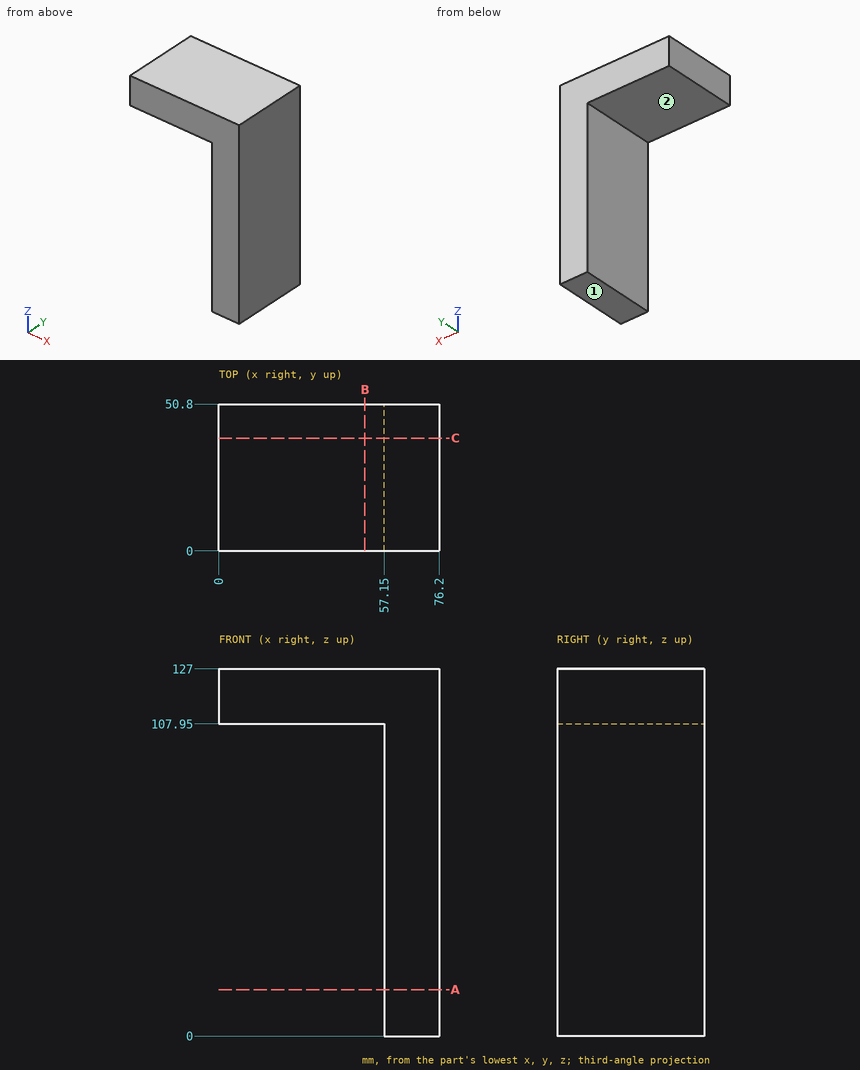
Answer from the drawing. Dimensions are ordinates in mm from the lowest x, y and z of the part. A direction names the side the tool comes from. Give positions to 0.01 mm unless a question says otherwise; leave off trailing zeros. Order: outer loops, then holes, each group sorted by start corner. A loop starts at its lowest first (then second) coordinate and runs counter-clockwise, first axis right, second up. Notation, with made-up numbers: (48.25, 43) -> (55.25, 43) arc R30 ccw to (55.25, 68) -> close; hole circle Ø2 at (73, 75.25). An arc over 180 degrees is marked (long way). One line per item, written item: value. Start each with the question number.
(1) The part is cut by section A-A (z = 16). Determine the outline of the cut face in (x, y), and give its area (3 significant figures).
(2) A tool of negligible diameter and unlimited length cuts with its end or side. For the marked faces 1 and 2, from which of +Z, -Z, +X, -X, +Y, -Y can it reach the whole face along a straight path? Write none if from no direction.
(3) Straight lines are drawn through the part: L1, parallel to X at y = 5, z = 89.5; L2, parallel to Z at x = 45, y = 8.5. For each, find the intervals that lie inside material, in ascending order.
(4) A flat-ended cylindrical pin translates along its axis: P1, Ø3, axis at y = 15.5, z = 17.5, coming from the -X side. Find the tip coordinate at first contact, or state that the pin passes through.
(5) The part is cut by section C-C (y = 39). Determine the outline of the cut face in (x, z), and give its area (3 significant figures).
(6) The part is cut by section B-B (x = 50.5). Determine the outline of the cut face in (y, z), and give its area (3 significant figures).
Taken from the geometry:
1. outline: (57.15, 0) -> (76.2, 0) -> (76.2, 50.8) -> (57.15, 50.8) -> close
1. area: 968 mm^2
2. face 1: -Z, +X, -X, +Y, -Y
2. face 2: -Z, -X, +Y, -Y
3. L1: 57.15 to 76.2
3. L2: 107.95 to 127
4. P1: x = 57.15
5. outline: (0, 107.95) -> (57.15, 107.95) -> (57.15, 0) -> (76.2, 0) -> (76.2, 127) -> (0, 127) -> close
5. area: 3,510 mm^2
6. outline: (0, 107.95) -> (50.8, 107.95) -> (50.8, 127) -> (0, 127) -> close
6. area: 968 mm^2
